Build history of the part. All positions in model axes, mm. Face numbers are marked on the shaded views. A direction names the side the tool comes from. Round coordinates to 2 decimals unless told otherwise and drop trailing zeros. Write each loop counter-clockwise with the first axis right and the second up, starting at its lowest first coordinate (ties: lowest second). Pieces come first, ordered by that corner, then holes.
Item 1: Band-saw the part on D-D, the plane y = 4. Write the cut outline in (x, z).
Item 2: Wall check: probe 1 along X at (y, z) = (1.3, 0); probe 2 along X at (y, z) = (5.5, 0); probe 3 along Y at (x, z) = (12.5, -5). Give the ranges that are in metal, low to high.
Item 3: Band-saw the part on C-C, the plane x = -11.5. Write the cut outline in (y, z).
Item 4: Band-saw the part on B-B, the plane x = 0. Write the cut outline in (y, z), then the cut area to 3 significant figures.
Item 5: Mould opens along X. For the marked faces 1, 2 and 3 say: +X half, -X half, draft (parallel to the pull), parting line (faces both ways), or undercut.
Item 6: Band-saw the part on A-A, the plane z = 0. Write the cut outline in (x, y).
Item 7: Drop flat-ended pins along their axis: pin 1 Ø4 at (x, y) = (3.5, 7) entering from +Z; pin 2 Ø1 at (y, z) = (2, 6.5) entering from -X; pin 3 Ø2.5 at (x, z) = (11.5, 0) entering from +Y; pin 4 Ø1.5 at (x, y) = (0.5, 7) entering from +Z. Give the stop position or say it passes through.
Item 8: 3-axis set-ups, long thin cutter, end or side, ignore diameter. For the marked faces 4 and 5: which of +Z, -Z, +X, -X, +Y, -Y reach the whole face in a straight line?
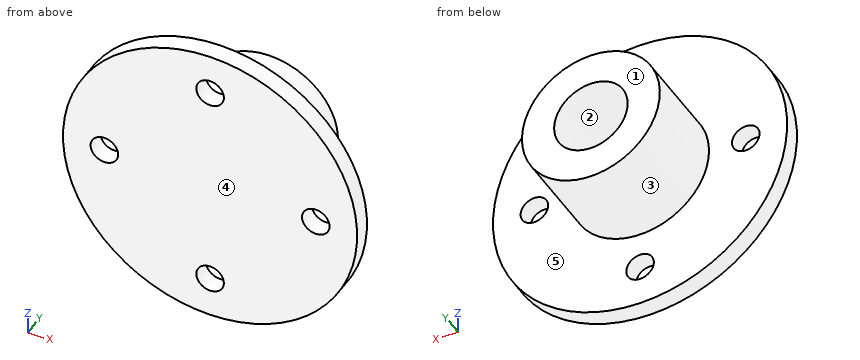
```python
from build123d import *

# Parameters (mm, degrees)
SKETCH_1_R          = 16
EXTRUDE_1_DEPTH     = 2
SKETCH_2_R          = 7.5
SKETCH_2_R_2        = 4
EXTRUDE_2_DEPTH     = 10
SKETCH_3_R          = 1.5
CUT_EXTRUDE_1_DEPTH = 10


with BuildPart() as part:
    # 草图1 → 凸台-拉伸1 (new body)
    with BuildSketch(Plane(origin=(0, 0, 0), x_dir=(1, 0, 0), z_dir=(0, 1, 0))):
        with Locations(Location((0, 0, 0), (0, 0, 270))):
            Circle(SKETCH_1_R)
    extrude(amount=EXTRUDE_1_DEPTH)

    # 草图2 → 凸台-拉伸2 (add)
    with BuildSketch(Plane(origin=(0, 2, 0), x_dir=(1, 0, 0), z_dir=(0, 1, 0))):
        with Locations(Location((0, 0, 0), (0, 0, 270))):
            Circle(SKETCH_2_R)
        with Locations(Location((0, 0, 0), (0, 0, 270))):
            Circle(SKETCH_2_R_2, mode=Mode.SUBTRACT)
    extrude(amount=EXTRUDE_2_DEPTH)

    # 草图3 → 切除-拉伸1 (cut)
    with BuildSketch(Plane(origin=(0, 2, 0), x_dir=(1, 0, 0), z_dir=(0, 1, 0))):
        with Locations(Location((-11.5, 0, 0), (0, 0, 270))):
            Circle(SKETCH_3_R)
        with Locations(Location((0, 11.5, 0), (0, 0, 270))):
            Circle(SKETCH_3_R)
        with Locations(Location((11.5, 0, 0), (0, 0, 270))):
            Circle(SKETCH_3_R)
        with Locations(Location((0, -11.5, 0), (0, 0, 270))):
            Circle(SKETCH_3_R)
    extrude(amount=-CUT_EXTRUDE_1_DEPTH, mode=Mode.SUBTRACT)


solid = part.part
```
Results:
1. outline: circle Ø15 at (0, 0); hole circle Ø8 at (0, 0)
2. probe 1: x = -16 to -13, -10 to 10, 13 to 16
2. probe 2: x = -7.5 to -4, 4 to 7.5
2. probe 3: y = 0 to 2
3. outline: (0, -11.12) - (2, -11.12) - (2, -1.5) - (0, -1.5) - close; (0, 1.5) - (2, 1.5) - (2, 11.12) - (0, 11.12) - close
4. outline: (0, -16) - (2, -16) - (2, -13) - (0, -13) - close; (0, -10) - (2, -10) - (2, -7.5) - (12, -7.5) - (12, -4) - (2, -4) - (2, 4) - (12, 4) - (12, 7.5) - (2, 7.5) - (2, 10) - (0, 10) - close; (0, 13) - (2, 13) - (2, 16) - (0, 16) - close
4. area: 122 mm2
5. face 1: draft
5. face 2: undercut
5. face 3: parting line
6. outline: (-16, 0) - (-13, 0) - (-13, 2) - (-16, 2) - close; (-10, 0) - (10, 0) - (10, 2) - (7.5, 2) - (7.5, 12) - (4, 12) - (4, 2) - (-4, 2) - (-4, 12) - (-7.5, 12) - (-7.5, 2) - (-10, 2) - close; (13, 0) - (16, 0) - (16, 2) - (13, 2) - close
7. pin 1: stops at z = 7.35
7. pin 2: stops at x = -14.83
7. pin 3: passes through
7. pin 4: stops at z = 7.5
8. face 4: +Z, -Z, +X, -X, -Y
8. face 5: +Y
